from build123d import *

# Parameters (mm, degrees)
Y_KSEKLIK_EKSTR_ZYON1_DEPTH = 9
IZIM2_R                     = 3.5
KES_EKSTR_ZYON1_DEPTH       = 1.5
IZIM3_R                     = 6
IZIM3_R_2                   = 4.5
KES_EKSTR_ZYON2_DEPTH       = 5
RADYUS1_R                   = 1


with BuildPart() as part:
    # Çizim1 → Yükseklik-Ekstrüzyon1 (new body)
    with BuildSketch(Plane(origin=(0, 0, 0), x_dir=(1, 0, 0), z_dir=(0, 1, 0))):
        with BuildLine():
            Line((3.16227766, 4.5), (-3.16227766, 4.5))
            ThreePointArc((-3.16227766, 4.5), (0, -5.5), (3.16227766, 4.5))
        make_face()
    extrude(amount=Y_KSEKLIK_EKSTR_ZYON1_DEPTH)

    # Çizim2 → Kes-Ekstrüzyon1 (cut)
    with BuildSketch(Plane.XZ):
        Circle(IZIM2_R)
    extrude(amount=-KES_EKSTR_ZYON1_DEPTH, mode=Mode.SUBTRACT)

    # Çizim3 → Kes-Ekstrüzyon2 (cut)
    with BuildSketch(Plane(origin=(0, 9, 0), x_dir=(1, 0, 0), z_dir=(0, 1, 0))):
        Circle(IZIM3_R)
        Circle(IZIM3_R_2, mode=Mode.SUBTRACT)
    extrude(amount=-KES_EKSTR_ZYON2_DEPTH, mode=Mode.SUBTRACT)

    # Radyus1
    radyus1_edges = [part.edges().sort_by_distance(p)[0] for p in [
        (-4.5, 9, 0),
    ]]
    fillet(radyus1_edges, radius=RADYUS1_R)


solid = part.part
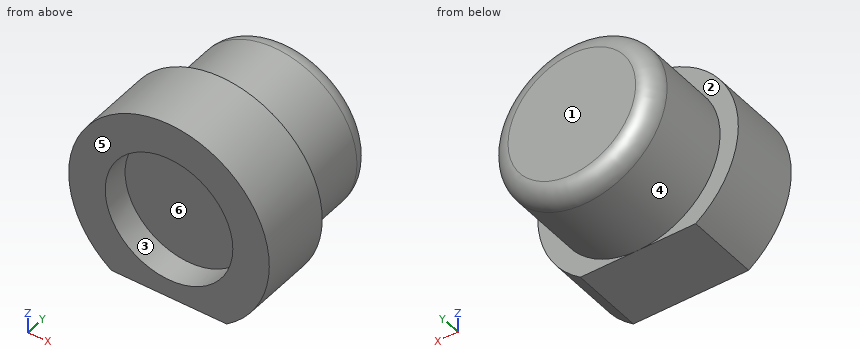
Verification items for the finished model (mm, model axes). Face numbers are marked on the shaded views. A direction names the side the tool comes from. Coordinates: 2 decimals unless noted, no trailing zeros. Order: outer loops, then holes, each group sorted by start corner. A loop starts at its lowest first (then second) coordinate and runs counter-clockwise, first axis right, second up. Notation, with made-up numbers: M -39,73.25 L 12,73.25 A17 ccw 12,81.25 Z; hole C -17.5,68.25 d8. An arc over 180 degrees is marked long. One line per item, written item: value. Start each with the question number.
Item 1: Access from +Z, -Z, +X, -X, +Y, -Y to the whole of each face (thin tool, end or side, straight path). Record for the marked faces 1 and 2.
Item 2: Sectioned sample at A-A on z = 0. Record the cut outline in (x, y).
Item 3: Sectioned sample at B-B on y = 7. Record the cut outline in (x, z), then the cut area to 3 significant figures.
Item 4: Depth check by flat-ended pin: P1, Ø2, axis at x = -0.5, z = 0.5, coming from the -Y side; P2, Ø4, axis at x = 1.5, y = 8, coming from the +Z side; P3, Ø4, axis at y = 3.5, z = -3.5, coming from the +X side. Enter the tip coordinate at first touch or a pass-through.
Item 5: Mould release check, pull along X, two halves, no side actions. Record for the marked faces 3, 4, 5 and 6: pulls with the +X half, pulls with the -X half, needs draft (parallel to the pull), parting line crosses it, or undercut.
Item 6: Thickness scan on probe 1 along Z at (x, y) = (0, 0.6); probe 2 along Y at (x, z) = (-4.5, 1.75); probe 3 along Y at (x, z) = (-1, 2). Record the ranges inside material, lowest first.
Item 7: Sectioned sample at C-C on z = 4.75. Record the cut outline in (x, y), then the cut area to 3 significant figures.
Calculated:
1. face 1: +Z, -Z, +X, -X, +Y
1. face 2: +Y
2. outline: M -5.5,0 L -3.5,0 L -3.5,1.5 L 3.5,1.5 L 3.5,0 L 5.5,0 L 5.5,4 L 4.5,4 L 4.5,8 A1 ccw 3.5,9 L -3.5,9 A1 ccw -4.5,8 L -4.5,4 L -5.5,4 Z
3. outline: C 0,0 d9
3. area: 63.6 mm^2
4. P1: y = 1.5
4. P2: z = 4.5
4. P3: x = 5.29
5. face 3: undercut
5. face 4: parting line crosses it
5. face 5: needs draft
5. face 6: undercut
6. probe 1: -4.5 to -3.5, 3.5 to 5.5
6. probe 2: 0 to 4
6. probe 3: 1.5 to 9
7. outline: M -2.77,0 L 2.77,0 L 2.77,4 L -2.77,4 Z
7. area: 22.2 mm^2
